```python
from build123d import *

# Parameters (mm, degrees)
SKETCH1_W           = 48.25
SKETCH1_H           = 48.25
SKETCH1_R           = 2.5
SKETCH1_R_2         = 4.125
BOSS_EXTRUDE1_DEPTH = 5


with BuildPart() as part:
    # Sketch1 → Boss-Extrude1 (new body)
    # profile 1 of 5: a face of its own
    with BuildSketch(Plane.XY):
        with Locations((24.125, 24.125)):
            Rectangle(SKETCH1_W, SKETCH1_H)
        with Locations((24.125, 24.125)):
            Circle(SKETCH1_R, mode=Mode.SUBTRACT)
        Polygon((34.895909278, 1.8), (30.666818556, 9.125), (34.895909278, 16.45), (43.354090722, 16.45), (47.583181444, 9.125), (43.354090722, 1.8), align=None, mode=Mode.SUBTRACT)
        Polygon((13.354090722, 1.8), (17.583181444, 9.125), (13.354090722, 16.45), (4.895909278, 16.45), (0.666818556, 9.125), (4.895909278, 1.8), align=None, mode=Mode.SUBTRACT)
        Polygon((34.895909278, 31.8), (43.354090722, 31.8), (47.583181444, 39.125), (43.354090722, 46.45), (34.895909278, 46.45), (30.666818556, 39.125), align=None, mode=Mode.SUBTRACT)
        Polygon((17.583181444, 39.125), (13.354090722, 31.8), (4.895909278, 31.8), (0.666818556, 39.125), (4.895909278, 46.45), (13.354090722, 46.45), align=None, mode=Mode.SUBTRACT)
    # profile 2 of 5: a face of its own
    with BuildSketch(Plane.XY):
        Polygon((30.666818556, 39.125), (34.895909278, 31.8), (43.354090722, 31.8), (47.583181444, 39.125), (43.354090722, 46.45), (34.895909278, 46.45), align=None)
        with Locations((39.125, 39.125)):
            Circle(SKETCH1_R_2, mode=Mode.SUBTRACT)
    # profile 3 of 5: a face of its own
    with BuildSketch(Plane.XY):
        Polygon((30.666818556, 9.125), (34.895909278, 16.45), (43.354090722, 16.45), (47.583181444, 9.125), (43.354090722, 1.8), (34.895909278, 1.8), align=None)
        with Locations((39.125, 9.125)):
            Circle(SKETCH1_R_2, mode=Mode.SUBTRACT)
    # profile 4 of 5: a face of its own
    with BuildSketch(Plane.XY):
        Polygon((4.895909278, 1.8), (13.354090722, 1.8), (17.583181444, 9.125), (13.354090722, 16.45), (4.895909278, 16.45), (0.666818556, 9.125), align=None)
        with Locations((9.125, 9.125)):
            Circle(SKETCH1_R_2, mode=Mode.SUBTRACT)
    # profile 5 of 5: a face of its own
    with BuildSketch(Plane.XY):
        Polygon((13.354090722, 31.8), (4.895909278, 31.8), (0.666818556, 39.125), (4.895909278, 46.45), (13.354090722, 46.45), (17.583181444, 39.125), align=None)
        with Locations((9.125, 39.125)):
            Circle(SKETCH1_R_2, mode=Mode.SUBTRACT)
    extrude(amount=BOSS_EXTRUDE1_DEPTH)


solid = part.part
```
Model file for the job. Use its own axes, mm. Coordinates: 2 decimals unless noted, no trailing zeros. Loops run counter-clockwise (first coordinate to the right, second up) from the corner with the lowest first, then second, coordinate; pieces in that order, holes last. Notation, with made-up numbers: M 48,13 L 82,13 A26 cw 82,49 Z; hole C 30,-32 d4. An arc over 180 degrees is marked long. Use CSV: the item, a comma, the result in double quotes. Start each with the question number.
1. Two-plate mould, pull along Y, no slides. Class faces 1 (the cylindrical face through (8.23, 5.1, 2.46)), 2 (the flat face through (48.25, 24, 2)), 3 (the flat face through (24, 0, 2)), 4 (the cylindrical face through (23.8, 26.604, 2.465)): pulls with the +Y half, pulls with the -Y half, needs draft (parallel to the pull), parting line crosses it, or undercut.
2. Band-saw the part on D-D, the plane z = 2. List the corners of the cut face in (x, y) (3 decimals), then the cut area to 3 significant figures.
3. Band-saw the part on A-A, the plane x = 12.5. List the corners of the cut face in (y, z), then the cut area to 3 significant figures.
4. Band-saw the part on C-C, the plane y = 23.5. List the corners of the cut face in (x, z).
5. Flat gauge pin, fed straight in: pin 1 (4 mm diameter, centred on x = 13, y = 5.5, fed in from -Z). Where does the tip first touch, or does it go through?
6. Band-saw the part on B-B, the plane y = 36. List the corners of the cut face in (x, z).
7. Probe probe 1 along Y at (x, z) = (9, 1.3); probe 2 along Y at (x, z) = (41.5, 3.95); probe 3 along X at (y, z) = (41, 1.8). List the from-to ranges inside material, lowest first. Write a range as [from, to].
Entries:
1,face 1,"undercut"
1,face 2,"needs draft"
1,face 3,"pulls with the -Y half"
1,face 4,"undercut"
2,outline,"M 0,0 L 48.25,0 L 48.25,48.25 L 0,48.25 Z; hole C 9.125,9.125 d8.25; hole C 9.125,39.125 d8.25; hole C 24.125,24.125 d5; hole C 39.125,9.125 d8.25; hole C 39.125,39.125 d8.25"
2,area,"2,090 mm2"
3,outline,"M 0,0 L 6.75,0 L 6.75,5 L 0,5 Z; M 11.5,0 L 36.75,0 L 36.75,5 L 11.5,5 Z; M 41.5,0 L 48.25,0 L 48.25,5 L 41.5,5 Z"
3,area,"194 mm2"
4,outline,"M 0,0 L 21.7,0 L 21.7,5 L 0,5 Z; M 26.55,0 L 48.25,0 L 48.25,5 L 26.55,5 Z"
5,pin 1,"stops at z = 0"
6,outline,"M 0,0 L 6.43,0 L 6.43,5 L 0,5 Z; M 11.82,0 L 36.43,0 L 36.43,5 L 11.82,5 Z; M 41.82,0 L 48.25,0 L 48.25,5 L 41.82,5 Z"
7,probe 1,"y = [0, 5], [13.25, 35], [43.25, 48.25]"
7,probe 2,"y = [0, 5.75], [12.5, 35.75], [42.5, 48.25]"
7,probe 3,"x = [0, 5.45], [12.8, 35.45], [42.8, 48.25]"
